Verification items for the finished model (mm, model axes). Face numbers are marked on the shaded views. A direction names the side the tool comes from. Coordinates: 2 decimals unless noted, no trailing zeros. Order: outer loops, then holes, each group sorted by start corner. A loop starts at its lowest first (then second) coordinate and runs counter-clockwise, first axis right, second up. Notation, with made-up numbers: M 41,-20 L 81,-20 A26 cw 81,12 Z; hole C 1,38.5 d4. An arc over 180 degrees is marked long. Return JSON: item names as keys, results as strings. Group by question number.
1. Section check B-B, the plane z = 1. Record the cut outline in (x, y), plus the area to 3 significant figures.
2. Mould release check, pull along Z, two halves, no side actions. Record for the marked faces 3, 4, 5 and 6: +Z half, -Z half, draft (parallel to the pull), parting line (faces both ways), or undercut.
3. Section check D-D, the plane y = 0.5. Record the cut outline in (x, z).
4. Section check C-C, the plane x = -9.5. Record the cut outline in (y, z), plus the area to 3 significant figures.
5. Gauge pin test, flat end, axial feed: pin 1 (6 mm diameter, centred on x = -7, z = 4, fed in from +Y). Record the tip position at first contact, or that the pin passes through.
6. Set-up check for the marked faces 1 and 2: record each of +Z, -Z, +X, -X, +Y, -Y from which the full face is reachable in a straight line by a thin tool's end or side.
7. Section check A-A, the plane y = -8.5. Record the cut outline in (x, z), plus the area to 3 significant figures.
8. Material ranges on line 1 along X through (y, z) = (-1.75, 4.75); line 2 along Z through (x, y) = (11.25, -10.5); line 3 along X through (y, z) = (5.75, 9.75), recorded low to high.
```python
from build123d import *

# Parameters (mm, degrees)
SKETCH1_W           = 26
SKETCH1_H           = 25
BOSS_EXTRUDE1_DEPTH = 10
SKETCH2_W           = 25
SKETCH2_H           = 9
CUT_EXTRUDE1_DEPTH  = 24
SKETCH3_W           = 9
SKETCH3_H           = 18.5
CUT_EXTRUDE2_DEPTH  = 5


with BuildPart() as part:
    # Sketch1 → Boss-Extrude1 (new body)
    with BuildSketch(Plane.XY):
        Rectangle(SKETCH1_W, SKETCH1_H)
    extrude(amount=BOSS_EXTRUDE1_DEPTH)

    # Sketch2 → Cut-Extrude1 (cut)
    with BuildSketch(Plane(origin=(0, 12.5, 0), x_dir=(1, 0, 0), z_dir=(0, 1, 0))):
        with Locations((0.067812243, -5.010506078)):
            Rectangle(SKETCH2_W, SKETCH2_H)
    extrude(amount=-CUT_EXTRUDE1_DEPTH, mode=Mode.SUBTRACT)

    # Sketch3 → Cut-Extrude2 (cut)
    with BuildSketch(Plane.XY.offset(10)):
        with Locations((0, 3.25)):
            Rectangle(SKETCH3_W, SKETCH3_H)
    extrude(amount=-CUT_EXTRUDE2_DEPTH, mode=Mode.SUBTRACT)


solid = part.part
```
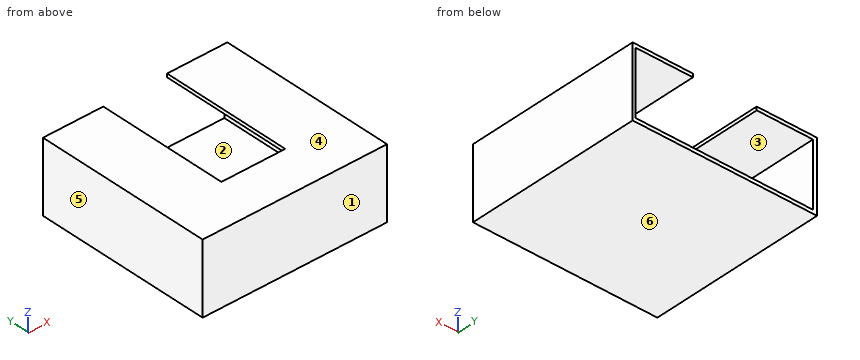
Answers follow:
{
 "1": {"outline": "M -13,-12.5 L 13,-12.5 L 13,12.5 L 12.57,12.5 L 12.57,-11.5 L -12.43,-11.5 L -12.43,12.5 L -13,12.5 Z", "area": "50.0 mm^2"},
 "2": {"face 3": "undercut", "face 4": "+Z half", "face 5": "draft", "face 6": "-Z half"},
 "3": {"outline": "M -13,0 L 13,0 L 13,10 L 4.5,10 L 4.5,9.51 L 12.57,9.51 L 12.57,0.51 L -12.43,0.51 L -12.43,9.51 L -4.5,9.51 L -4.5,10 L -13,10 Z"},
 "4": {"outline": "M -12.5,0 L 12.5,0 L 12.5,0.51 L -11.5,0.51 L -11.5,9.51 L 12.5,9.51 L 12.5,10 L -12.5,10 Z", "area": "34.0 mm^2"},
 "5": {"pin 1": "y = -11.5"},
 "6": {"face 1": "+Z, -Z, +X, -X, -Y", "face 2": "+Y"},
 "7": {"outline": "M -13,0 L 13,0 L 13,10 L -13,10 Z; hole M -12.43,0.51 L 12.57,0.51 L 12.57,9.51 L -12.43,9.51 Z", "area": "35.0 mm^2"},
 "8": {"line 1": "-13 to -12.43, 12.57 to 13", "line 2": "0 to 0.51, 9.51 to 10", "line 3": "-13 to -4.5, 4.5 to 13"}
}
